Source: three-view drawing plus pictorial views. Frame: mm from the lowest corner of the part. Give positions to 0.01 mm unless a question says otherwise; leave off trailing zeros. Order: outer loops, then holes, each group sorted by start corner. A loop starts at its lowest first (then second) coordinate and runs counter-clockwise, first axis right, second up.
1) Material intervals for line 1 (Y direction, x = 80, z = 0.75); line 2 (Y direction, x = 45, z = 1.2); line 3 (Y direction, x = 43, z = 0.5), sorted ascending.
2) Section D-D, the plane x = 45. Return loops of the section in (y, z), plus the area to 3 significant figures.
3) First-contact query: P1, Ø1.5, axis at x = 37, y = 14.5, coming from the -Z side. Flat tip, straight axial feed; report the tip coordinate or a pass-through.
4) Section C-C, the plane z = 0.5. Return loops of the section in (x, y).
5) Section A-A, the plane y = 60. Return loops of the section in (x, z), plus the area to 3 significant figures.
6) Section B-B, the plane x = 10. Return loops of the section in (y, z), plus the area to 3 significant figures.
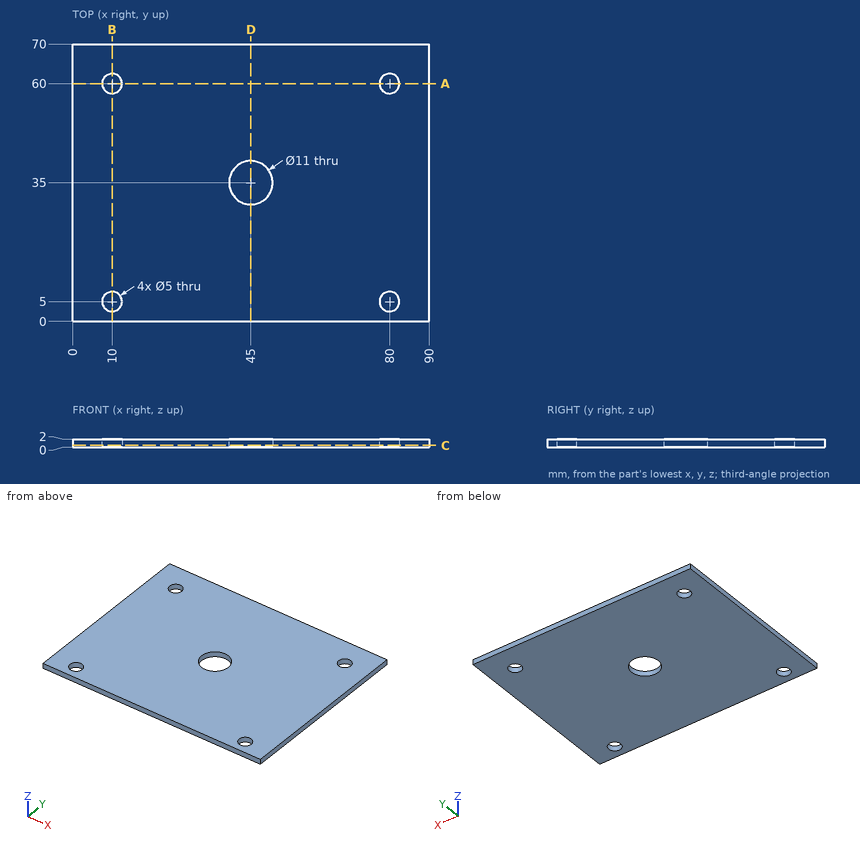
From the geometry:
1. line 1: y = 0 to 2.5, 7.5 to 57.5, 62.5 to 70
1. line 2: y = 0 to 29.5, 40.5 to 70
1. line 3: y = 0 to 29.88, 40.12 to 70
2. outline: (0, 0) - (29.5, 0) - (29.5, 2) - (0, 2) - close; (40.5, 0) - (70, 0) - (70, 2) - (40.5, 2) - close
2. area: 118 mm2
3. P1: stops at z = 0
4. outline: (0, 0) - (90, 0) - (90, 70) - (0, 70) - close; hole circle Ø5 at (10, 5); hole circle Ø5 at (10, 60); hole circle Ø11 at (45, 35); hole circle Ø5 at (80, 5); hole circle Ø5 at (80, 60)
5. outline: (0, 0) - (7.5, 0) - (7.5, 2) - (0, 2) - close; (12.5, 0) - (77.5, 0) - (77.5, 2) - (12.5, 2) - close; (82.5, 0) - (90, 0) - (90, 2) - (82.5, 2) - close
5. area: 160 mm2
6. outline: (0, 0) - (2.5, 0) - (2.5, 2) - (0, 2) - close; (7.5, 0) - (57.5, 0) - (57.5, 2) - (7.5, 2) - close; (62.5, 0) - (70, 0) - (70, 2) - (62.5, 2) - close
6. area: 120 mm2
